Part model, mm, in its own coordinate system. A direction names the side the tool comes from. Coordinates: 2 decimals unless noted, no trailing zeros. Loops run counter-clockwise (first coordinate to the right, second up) from the corner with the lowest first, then second, coordinate; pieces in that order, holes last. Notation, with made-up numbers: M 8,87.5 L 31,87.5 A17 ccw 31,108.5 Z; hole C 52.5,39 d4. An arc over 180 degrees is marked long. Use a Markdown table: item, result. Add a question column.
1) Band-saw the part on A-A (x = 0). List the corners of the cut face in (y, z).
2) Wall check: probe 1 along Z at (x, y) = (0, 7.5); probe 2 along Z at (x, y) = (5.5, 10.25); probe 3 along Y at (x, z) = (-18, -3.5). Give the ranges that are in metal, low to high. Write a range as from..to.
3) Band-saw the part on D-D (x = -8). List the corners of the cut face in (y, z), plus the area to 3 significant figures.
4) Tool access for faces 1 (the flat face through (0, 0, 0)), 2 (the flat face through (4, 3, 14)): list every direction of +Z, -Z, +X, -X, +Y, -Y with a clear straight run to the whole face (end or side of a thin tool).
5) Pull direction Z, two halves, no side cores. Call faces 3 (the cylindrical face through (12.932, 4.479, 5.362)), 4 (the cylindrical face through (8.86, 7.89, 0.27)), 5 (the flat face through (0, 16, 0)): released by +Z, released by -Z, zero draft, split by the parting line, or undercut.
6) Band-saw the part on B-B (z = 0). List the corners of the cut face in (x, y), plus the area to 3 significant figures.
7) Band-saw the part on C-C (z = -8). List the corners of the cut face in (x, y), plus the area to 3 significant figures.
8) Pin check, flat tips, straight feed: pin 1 Ø2.5 at (x, z) = (8, 0) entering from +Y; pin 2 Ø8 at (y, z) = (9, -7) entering from +X; pin 3 Ø1.6 at (x, z) = (0, -8) entering from -Y. Stop position of each tip, or through.
from build123d import *

# Parameters (mm, degrees)
SKETCH_1_R          = 21
EXTRUDE_1_DEPTH     = 3
SKETCH_2_R          = 10
EXTRUDE_2_DEPTH     = 13
SKETCH_3_R          = 14
EXTRUDE_3_DEPTH     = 3
SKETCH_4_R          = 0.9
CUT_EXTRUDE_1_DEPTH = 16


with BuildPart() as part:
    # 스케치1 → 보스-돌출1 (new body)
    with BuildSketch(Plane(origin=(0, 0, 0), x_dir=(1, 0, 0), z_dir=(0, 1, 0))):
        Circle(SKETCH_1_R)
    extrude(amount=EXTRUDE_1_DEPTH)

    # 스케치2 → 보스-돌출2 (add)
    with BuildSketch(Plane(origin=(0, 3, 0), x_dir=(1, 0, 0), z_dir=(0, 1, 0))):
        Circle(SKETCH_2_R)
    extrude(amount=EXTRUDE_2_DEPTH)

    # 스케치3 → 보스-돌출3 (add)
    with BuildSketch(Plane(origin=(0, 3, 0), x_dir=(1, 0, 0), z_dir=(0, 1, 0))):
        Circle(SKETCH_3_R)
    extrude(amount=EXTRUDE_3_DEPTH)

    # 스케치4 → 컷-돌출1 (cut)
    with BuildSketch(Plane.XZ):
        with Locations((8, 0)):
            Circle(SKETCH_4_R)
        with Locations((5.656854249, -5.656854249)):
            Circle(SKETCH_4_R)
        with Locations((5.656854249, 5.656854249)):
            Circle(SKETCH_4_R)
        with Locations((0, 8)):
            Circle(SKETCH_4_R)
        with Locations((-5.656854249, 5.656854249)):
            Circle(SKETCH_4_R)
        with Locations((0, -8)):
            Circle(SKETCH_4_R)
        with Locations((-5.656854249, -5.656854249)):
            Circle(SKETCH_4_R)
        with Locations((-8, 0)):
            Circle(SKETCH_4_R)
    extrude(amount=-CUT_EXTRUDE_1_DEPTH, mode=Mode.SUBTRACT)


solid = part.part
Entries:
| question | item | result |
|---|---|---|
| 1 | outline | M 0,-21 L 3,-21 L 3,-14 L 6,-14 L 6,-10 L 16,-10 L 16,-8.9 L 0,-8.9 Z; M 0,-7.1 L 16,-7.1 L 16,7.1 L 0,7.1 Z; M 0,8.9 L 16,8.9 L 16,10 L 6,10 L 6,14 L 3,14 L 3,21 L 0,21 Z |
| 2 | probe 1 | -10..-8.9, -7.1..7.1, 8.9..10 |
| 2 | probe 2 | -8.35..-6.54, -4.77..4.77, 6.54..8.35 |
| 2 | probe 3 | 0..3 |
| 3 | outline | M 0,-19.42 L 3,-19.42 L 3,-11.49 L 6,-11.49 L 6,-6 L 16,-6 L 16,-0.9 L 0,-0.9 Z; M 0,0.9 L 16,0.9 L 16,6 L 6,6 L 6,11.49 L 3,11.49 L 3,19.42 L 0,19.42 Z |
| 3 | area | 277 mm2 |
| 4 | face 1 | +Z, -Z, +X, -X, -Y |
| 4 | face 2 | +Y |
| 5 | face 3 | split by the parting line |
| 5 | face 4 | undercut |
| 5 | face 5 | zero draft |
| 6 | outline | M -21,0 L -8.9,0 L -8.9,16 L -10,16 L -10,6 L -14,6 L -14,3 L -21,3 Z; M -7.1,0 L 7.1,0 L 7.1,16 L -7.1,16 Z; M 8.9,0 L 21,0 L 21,3 L 14,3 L 14,6 L 10,6 L 10,16 L 8.9,16 Z |
| 6 | area | 352 mm2 |
| 7 | outline | M -19.42,0 L -0.9,0 L -0.9,16 L -6,16 L -6,6 L -11.49,6 L -11.49,3 L -19.42,3 Z; M 0.9,0 L 19.42,0 L 19.42,3 L 11.49,3 L 11.49,6 L 6,6 L 6,16 L 0.9,16 Z |
| 7 | area | 277 mm2 |
| 8 | pin 1 | y = 16 |
| 8 | pin 2 | x = 13.31 |
| 8 | pin 3 | through |
